Geometry: see drawing. Coordinates: mm, zero at the bounding-box minimum. Round coordinates to 2 decimals unless told otherwise and drop trailing zeros. Loops run counter-clockwise (first coordinate to the right, second up) from the corner with the lowest first, then second, coordinate; pieces in that order, holes last. Notation, with made-up numbers: (-37, -34) -> (4, -34) arc R26 cw to (4, 1) -> close; hole circle Ø10 at (-22.5, 59.25). An arc over 180 degrees is marked (long way). Write item = value, one per line.
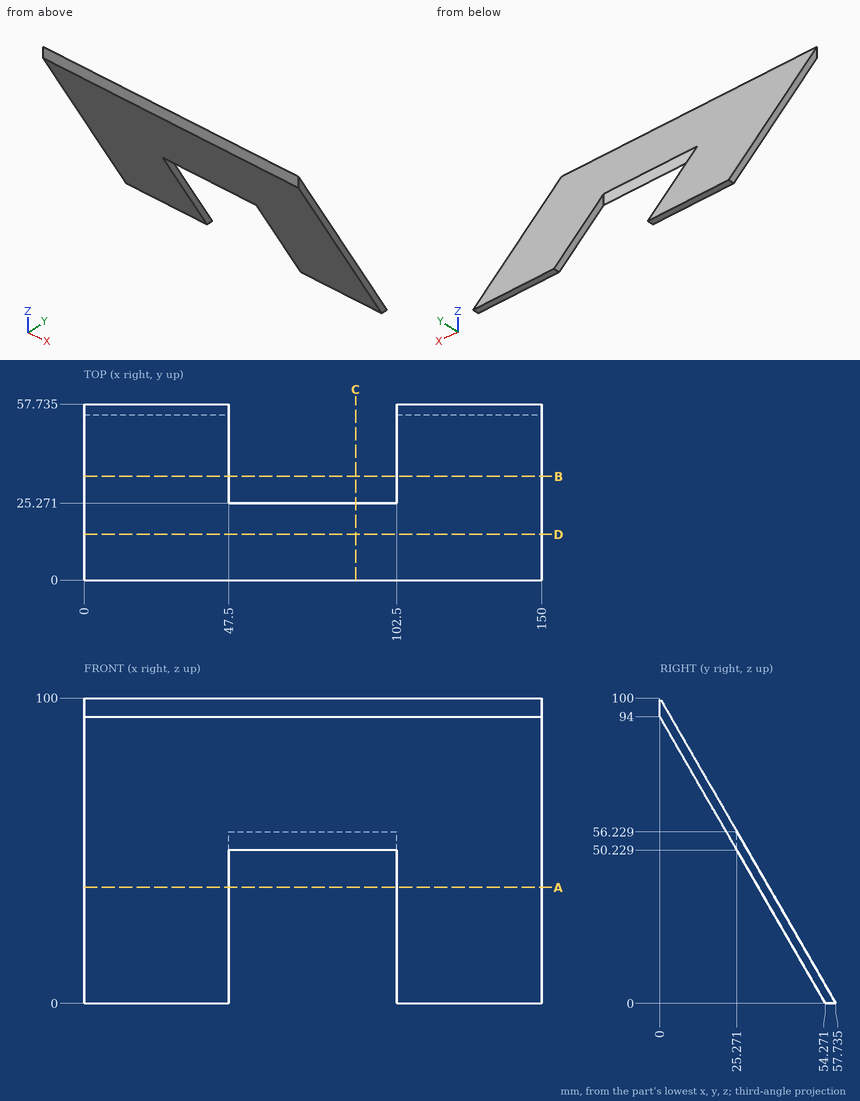
1. Section query B-B (y = 34). Return the cut outline in (x, z).
Evaluation:
outline = (0, 35.11) -> (47.5, 35.11) -> (47.5, 41.11) -> (0, 41.11) -> close; (102.5, 35.11) -> (150, 35.11) -> (150, 41.11) -> (102.5, 41.11) -> close
2. Section query C-C (x = 89). Return the cut outline in (y, z), then the cut area to 3 significant figures.
Evaluation:
outline = (0, 94) -> (25.27, 50.23) -> (25.27, 56.23) -> (0, 100) -> close
area = 152 mm²
3. Line query: probe 1 along X at (y, z) = (39, 30); probe 2 along Y at (x, z) = (136, 39.5) (1 decimal); probe 3 along Z at (x, y) = (44, 22) (1 decimal). Output: solid intervals per line, ascending. Write a range as from..to.
Evaluation:
probe_1 = 0..47.5, 102.5..150
probe_2 = 31.5..34.9
probe_3 = 55.9..61.9
4. Section query A-A (z = 38). Return the cut outline in (x, y) (1 decimal).
Evaluation:
outline = (0, 32.3) -> (47.5, 32.3) -> (47.5, 35.8) -> (0, 35.8) -> close; (102.5, 32.3) -> (150, 32.3) -> (150, 35.8) -> (102.5, 35.8) -> close
5. Section query D-D (y = 15). Return the cut outline in (x, z), then the cut area to 3 significant figures.
Evaluation:
outline = (0, 68.02) -> (150, 68.02) -> (150, 74.02) -> (0, 74.02) -> close
area = 900 mm²
6. Contact query for flat-ended pins moving along their axis: pin 1 Ø1 at (x, z) = (18, 41) entering from -Y; pin 2 Ø3 at (x, z) = (53.5, 67.5) entering from +Y; pin 3 Ø12 at (x, z) = (134, 80.5) entering from -Y. Output: stop coordinate, or through.
Evaluation:
pin_1 = 30.31
pin_2 = 19.63
pin_3 = 4.33
